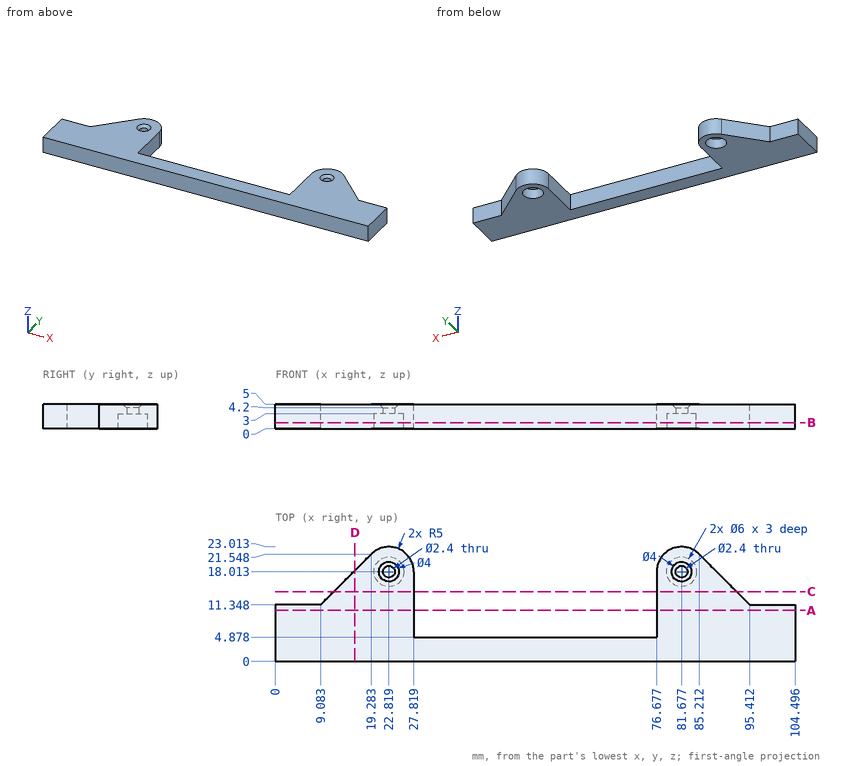
Part print with two shaded views. Sizes in mm from the minimum x, y, z corner. Round coordinates to 2 decimals unless told otherwise and drop trailing zeros. Order: outer loops, then holes, each group sorted by start corner. A loop starts at its lowest first (then second) coordinate and runs counter-clockwise, first axis right, second up. Notation, with made-up numbers: (15.25, -39) - (71.25, -39) arc R27 cw to (71.25, 0) - close; hole circle Ø4 at (-17.75, -5.5). An arc over 180 degrees is marked (long way). Answer in a Markdown table with one row per item. Add a question column.
(1) Band-saw the part on B-B on z = 1.25. List the corners of the cut face in (x, y) (1 decimal), and give its area (3 significant figures).
(2) Drop flat-ended pins along their axis: pin 1 Ø1.8 at (x, y) = (82.5, 18) entering from -Z; pin 2 Ø2.5 at (x, z) = (63, 2.5) entering from +Y; pin 3 Ø1.5 at (y, z) = (14, 2) entering from +X. Give the stop position or say it passes through.
(3) Probe L1, parallel to X at y = 9.75, z = 0.85 (1 decimal); L2, parallel to X at y = 19, z = 4.2 (1 decimal); L3, parallel to Y at x = 36, z = 3.1. List the from-to ranges inside material, lowest first. Write a range as [from, to].
(4) Band-saw the part on A-A on y = 10.25. List the corners of the cut face in (x, z) (1 decimal), and give its area (3 significant figures).
(5) Band-saw the part on C-C on y = 14. List the corners of the cut face in (x, z) (1 decimal), and give its area (3 significant figures).
(6) Band-saw the part on D-D on x = 16. List the corners of the cut face in (y, z) (1 decimal).
Data:
| question | item | result |
|---|---|---|
| 1 | outline | (0, 0) - (104.5, 0) - (104.5, 11.3) - (95.4, 11.3) - (85.2, 21.5) arc R5 ccw to (76.7, 18) - (76.7, 4.9) - (27.8, 4.9) - (27.8, 18) arc R5 ccw to (19.3, 21.5) - (9.1, 11.3) - (0, 11.3) - close; hole circle Ø6 at (22.8, 18); hole circle Ø6 at (81.7, 18) |
| 1 | area | 1,100 mm^2 |
| 2 | pin 1 | stops at z = 3 |
| 2 | pin 2 | stops at y = 4.88 |
| 2 | pin 3 | stops at x = 93.51 |
| 3 | L1 | x = [0, 27.8], [76.7, 104.5] |
| 3 | L2 | x = [16.7, 22.1], [23.5, 27.7], [76.8, 81], [82.4, 87.8] |
| 3 | L3 | y = [0, 4.88] |
| 4 | outline | (0, 0) - (27.8, 0) - (27.8, 5) - (0, 5) - close; (76.7, 0) - (104.5, 0) - (104.5, 5) - (76.7, 5) - close |
| 4 | area | 278 mm^2 |
| 5 | outline | (11.7, 0) - (27.8, 0) - (27.8, 5) - (11.7, 5) - close; (76.7, 0) - (92.8, 0) - (92.8, 5) - (76.7, 5) - close |
| 5 | area | 161 mm^2 |
| 6 | outline | (0, 0) - (18.3, 0) - (18.3, 5) - (0, 5) - close |
